For this review, take the finished solid that the model builds, in its own axes (mm). Face numbers are marked on the shaded views. A direction names the side the tool comes from. Round coordinates to 2 decimals unless told otherwise and drop trailing zeros. Order: outer loops, then holes, each group sorted by start corner. A loop starts at its lowest first (then second) coordinate and runs counter-clockwise, first axis right, second up. Notation, with made-up numbers: (48, -10) - (62, -10) arc R36 cw to (62, 25) - close; hole circle Ø10 at (4, 33). An arc over 180 degrees is marked (long way). One line per item, written item: value.
Autodesk Inventor part; units mm, degrees
ref_plane "YZ Plane" through (0, 0, 0) normal (1, 0, 0) x (0, 1, 0)
ref_plane "XZ Plane" through (0, 0, 0) normal (0, 1, 0) x (-1, 0, 0)
ref_plane "XY Plane" through (0, 0, 0) normal (0, 0, 1) x (1, 0, 0)
sketch "Sketch1" plane through (0, 0, 0) normal (0, 0, 1) x (1, 0, 0)
  circle A0 centre (0, 0) radius 1.6964
  line L0 (0, 0) -> (1.6964, 0)
  line L1 (1.6964, 0) -> (1.6964, 1.8999)
  line L2 (1.6964, 1.8999) -> (0, 1.8999)
  line L3 (0, 1.8999) -> (0, 0)
  line L4 (0, 0) -> (-1.6964, 0)
  line L5 (-1.6964, 0) -> (-1.6964, 1.8999)
  line L6 (-1.6964, 1.8999) -> (0, 1.8999)
  line L7 (0, 1.8999) -> (0, 0)
  point P0 (0, 1.6964)
extrude "Extrusion1" add sketch "Sketch1" along normal blind 20 contours L4 L0 A0 | A0 L3 L4 | L0 L3 A0
extrude "Extrusion2" add sketch "Sketch1" along normal blind 10 contours L5 L6 L3 A0 | A0 L3 L2 L1
properties part number "Sensor"
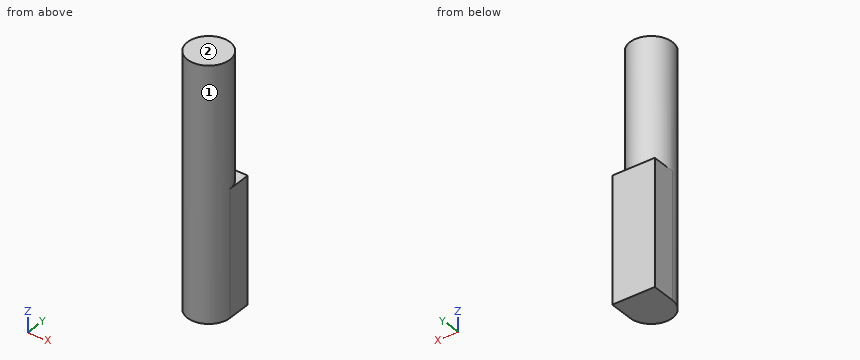
Item 1: Take a section at A-A (x = 0). Write out the cut boundary in (y, z).
Returned:
outline: (-1.7, 0) - (1.9, 0) - (1.9, 10) - (1.7, 10) - (1.7, 20) - (-1.7, 20) - close
Item 2: For P1, Ø1, axis at x = -1, z = 17, coming from the -Y side, flat-tipped, find the tip position at first contact; note if it passes through.
Returned:
P1: y = -1.62
Item 3: Wall thickness on line 1 (Z direction, x = -0.9, y = 1.55); line 2 (Y direction, x = 0, z = 13.5); line 3 (X direction, y = -0.85, z = 5): over which ranges is each line inside the solid? List them lowest first.
Returned:
line 1: 0 to 10
line 2: -1.7 to 1.7
line 3: -1.47 to 1.47
Item 4: Take a section at C-C (z = 3.5). Write out the cut boundary in (x, y).
Returned:
outline: (-1.7, 0) arc R1.7 ccw to (1.7, 0) - (1.7, 1.9) - (-1.7, 1.9) - close
Item 5: Take a section at D-D (x = 0.8). Write out the cut boundary in (y, z), plus the area to 3 significant figures.
Returned:
outline: (-1.5, 0) - (1.9, 0) - (1.9, 10) - (1.5, 10) - (1.5, 20) - (-1.5, 20) - close
area: 63.9 mm^2
Item 6: Machinability: for the marked faces 1 and 2, which of the approach directions +Z, -Z, +X, -X, +Y, -Y give a long, thin tool a straight path to every point of the face, cutting with its end or side? Answer none if there is none.
Returned:
face 1: +Z
face 2: +Z, +X, -X, +Y, -Y
Item 7: Take a section at B-B (y = 0.8). Write out the cut boundary in (x, z), plus the area to 3 significant figures.
Returned:
outline: (-1.7, 0) - (1.7, 0) - (1.7, 10) - (1.5, 10) - (1.5, 20) - (-1.5, 20) - (-1.5, 10) - (-1.7, 10) - close
area: 63.8 mm^2
